Verification items for the finished model (mm, model axes). A direction names the side the tool comes from. Round coordinates to 2 decimals unless told otherwise and drop trailing zeros. Order: outer loops, then holes, each group sorted by start corner. A loop starts at its lowest first (then second) coordinate and runs counter-clockwise, first axis right, second up. Notation, with made-up numbers: (1.5, 51.5) -> (39.5, 51.5) arc R18 cw to (39.5, 78.5) -> close; hole circle Ø4 at (80, -16). An arc over 180 degrees is marked (long way). Write item = value, one per line. Start each with the question number.
from build123d import *

# Parameters (mm, degrees)
SKETCH004_R       = 2.125
PAD001_DEPTH      = 5
PAD002_DEPTH      = 1.5
PAD003_DEPTH      = 8.5
PAD_DEPTH         = 53
SKETCH001_W       = 43
SKETCH001_H       = 38.1
POCKET_DEPTH      = 19.351
POCKET_DEPTH_BACK = 13.683516
CHAMFER_1_SIZE2   = 6
CHAMFER_1_SIZE    = 18.75
CHAMFER_2_SIZE2   = 6
CHAMFER_2_SIZE    = 18.75
FILLET_R          = 10
SKETCH002_W       = 60
SKETCH002_H       = 13
POCKET001_DEPTH   = 1.4
CHAMFER001_SIZE   = 2


with BuildPart() as body001:
    # Sketch004 → Pad001 (new body)
    with BuildSketch(Plane.XY):
        Polygon((0, 0), (0, 10), (53, 10), (53, -10), (0, -10), align=None)
        with Locations((44.5, 0)):
            Circle(SKETCH004_R, mode=Mode.SUBTRACT)
    extrude(amount=-PAD001_DEPTH)

    # Sketch005 (on Face3 of Pad001) → Pad002 (join)
    with BuildSketch(Plane.YZ.offset(53)):
        Polygon((-10, 45), (10, 0), (-10, 0), (-10, -5), (-13.6, 3.691169), (-13.6, 45), align=None)
    extrude(amount=-PAD002_DEPTH)

    # Sketch006 (on Face9 of Pad002) → Pad003 (join)
    with BuildSketch(Plane(origin=(51.5, 0, 0), x_dir=(0, -1, 0), z_dir=(-1, 0, 0))):
        Polygon((10, 35), (10, -5), (13.6, 3.691169), (13.6, 29), (11, 29), (11, 35), align=None)
    extrude(amount=PAD003_DEPTH)


with BuildPart() as body001_1:
    # Body001 placement: moved
    add(body001.part.moved(Location((0, 29.35, 0))))


with BuildPart() as body002:
    # Sketch → Pad (new body)
    with BuildSketch(Plane.YZ):
        with BuildLine():
            ThreePointArc((15.75, 71.85), (6.027264, 86.401103), (-11.136932, 82.986932))
            Line((-11.136932, 82.986932), (-13.682516, 85.532516))
            ThreePointArc((19.35, 71.85), (7.404924, 89.727069), (-13.682516, 85.532516))
            Line((19.35, 71.85), (19.35, 19.35))
            ThreePointArc((-13.682516, 5.667484), (7.404924, 1.472931), (19.35, 19.35))
            Line((-11.136932, 8.213068), (-13.682516, 5.667484))
            ThreePointArc((-11.136932, 8.213068), (6.027264, 4.798897), (15.75, 19.35))
            Line((15.75, 71.85), (15.75, 19.35))
        make_face()
    extrude(amount=PAD_DEPTH)

    # Sketch001 → Pocket (cut, two sides)
    with BuildSketch(Plane.XZ) as pocket_sk:
        with Locations((21.5, 19.05)):
            Rectangle(SKETCH001_W, SKETCH001_H)
        with Locations((21.5, 72.15)):
            Rectangle(SKETCH001_W, SKETCH001_H)
    extrude(amount=-POCKET_DEPTH, mode=Mode.SUBTRACT)
    extrude(pocket_sk.sketch, amount=POCKET_DEPTH_BACK, mode=Mode.SUBTRACT)

    # Chamfer 1
    chamfer_1_edges = [body002.edges().sort_by_distance(p)[0] for p in [
        (43, 17.55, 53.1),
    ]]
    chamfer_1_side = body002.faces().sort_by_distance((43, 16.254258, 62.475))[0]
    chamfer(chamfer_1_edges, length=CHAMFER_1_SIZE, length2=CHAMFER_1_SIZE2, reference=chamfer_1_side)

    # Chamfer 2
    chamfer_2_edges = [body002.edges().sort_by_distance(p)[0] for p in [
        (43, 17.55, 38.1),
    ]]
    chamfer_2_side = body002.faces().sort_by_distance((43, -7.211953, 1.938804))[0]
    chamfer(chamfer_2_edges, length=CHAMFER_2_SIZE, length2=CHAMFER_2_SIZE2, reference=chamfer_2_side)

    # Fillet
    fillet_edges = [body002.edges().sort_by_distance(p)[0] for p in [
        (37, 17.55, 38.1),
        (43, 17.55, 19.35),
        (37, 17.55, 53.1),
        (43, 17.55, 71.85),
    ]]
    fillet(fillet_edges, radius=FILLET_R)

    # Sketch002 → Pocket001 (cut, symmetric)
    with BuildSketch(Plane(origin=(0, 15.75, 0), x_dir=(0, 0, -1), z_dir=(0, -1, 0))):
        with Locations((-44, 39.5)):
            Rectangle(SKETCH002_W, SKETCH002_H)
    extrude(amount=POCKET001_DEPTH, both=True, mode=Mode.SUBTRACT)

    # Chamfer001
    chamfer001_edges = [body002.edges().sort_by_distance(p)[0] for p in [
        (43, -12.409724, 6.940276),
        (53, -12.409724, 6.940276),
        (43, -12.409724, 84.259724),
        (53, -12.409724, 84.259724),
    ]]
    chamfer(chamfer001_edges, length=CHAMFER001_SIZE)


with BuildPart() as body002_1:
    # Body placement: moved
    add(body002.part.moved(Location((0, 0, 15))))

    # Connect: union Body001
    add(body001_1.part)


with BuildPart() as part_mirroring:
    # Part__Mirroring: instance of Body002
    add(body002_1.part.mirror(Plane(origin=(0, 0, 0), x_dir=(0, -1, 0), z_dir=(1, 0, 0))))


solid = part_mirroring.part
(1) Cross-section at D-D (y = -8). Enter the section's corners in (x, z).
(2) Scan lines: line 1 along Z through (x, y) = (-31, 28.5); line 2 along Y through (x, z) = (-20, 54); line 3 along Z through (x, y) = (-48, 9.5). Record each from-to range of solid material in increasing order. Write a range as from..to.
(3) Cross-section at A-A (y = 29.35). Enter the section's corners in (x, z) (3 decimals).
(4) Draft check along Z on faces 4 (the flat face through (-47.96, -12.39, 21.96)), 5 (the flat face through (-27, 29, -5)), 6 (the flat face through (-26, 39.35, -2)). Enter one of: +Z half, -Z half, draft (parallel to the pull), parting line (faces both ways), or undercut.
(5) Cross-section at C-C (z = 58). Enter the section's corners in (x, y).
(6) Depth check by flat-ended pin: pin 1 (4 mm diameter, centred on x = -13, y = 18, fed in from +Z); pin 2 (10 mm diameter, centred on y = 29.5, z = 13.5, fed in from +X); pin 3 (1.5 mm diameter, centred on x = -26.5, z = -3, fed in from -Y). Enter the tip coordinate at first touch or a pass-through.
(7) Set-up check for faces 1 (the flat face through (-22, 19.35, -2)), 2 (the cylindrical face through (-47.93, 5.786, 19.701)), 3 (the flat face through (-51.5, 25, 13)): record each of +Z, -Z, +X, -X, +Y, -Y from which the full face is reachable in a straight line by a thin tool's end or side.
(8) Cross-section at B-B (x = -37.5). Enter the section's corners in (y, z).
Outcome:
q1.outline = (-53, 16.73) -> (-43, 16.73) -> (-43, 20.78) -> (-53, 20.78) -> close; (-53, 100.42) -> (-43, 100.42) -> (-43, 104.47) -> (-53, 104.47) -> close
q2.line_1 = -5..0
q2.line_2 = 15.75..19.35
q2.line_3 = 17.49..21.79, 99.41..103.71
q3.outline = (-53, -5) -> (-46.625, -5) -> (-46.625, 0) -> (-51.5, 0) -> (-51.5, 22.5) -> (-53, 22.5) -> close; (-42.375, -5) -> (0, -5) -> (0, 0) -> (-42.375, 0) -> close
q4.face_4 = undercut
q4.face_5 = -Z half
q4.face_6 = draft
q5.outline = (-53, 15.75) -> (-46, 15.75) -> (-46, 17.15) -> (-33, 17.15) -> (-33, 15.75) -> (0, 15.75) -> (0, 19.35) -> (-53, 19.35) -> close
q6.pin_1 = 68.1
q6.pin_2 = -51.5
q6.pin_3 = 19.35
q7.face_1 = -Z, +X, -Y
q7.face_2 = +X, -X
q7.face_3 = +Z, +X, +Y
q8.outline = (17.15, 49.36) -> (19.35, 49.36) -> (19.35, 71.84) -> (17.15, 71.84) -> close; (19.35, -5) -> (39.35, -5) -> (39.35, 0) -> (19.35, 0) -> close
